```python
from build123d import *

# Parameters (mm, degrees)
F1_DEPTH = 14.37
F0_R     = 2
F2_DEPTH = 7.185
F3_DEPTH = 14.37


with BuildPart() as f1:
    # F0 (on Front) → F1 (new body)
    with BuildSketch(Plane.XZ):
        with BuildLine():
            Line((3.9000000034, 5.6), (2.8, 5.6))
            ThreePointArc((2.8, 5.6), (4.7798989873, 4.7798989873), (5.6, 2.8))
            ThreePointArc((5.6, 2.8), (6.0135800872, 1.3354181484), (7.1321428571, 0.3034947896))
            ThreePointArc((7.1321428571, 0.3034947896), (7.7481620558, 0.0769305381), (8.4, 0))
            Line((8.4, 0), (31.6, 0))
            ThreePointArc((31.6, 0), (32.2518379442, 0.0769305381), (32.8678571429, 0.3034947896))
            ThreePointArc((32.8678571429, 0.3034947896), (33.9864199128, 1.3354181484), (34.4, 2.8))
            ThreePointArc((34.4, 2.8), (35.2201010127, 4.7798989873), (37.2, 5.6))
            Line((37.2, 5.6), (37.2, 6.7))
            ThreePointArc((37.2, 6.7), (36.8778174593, 5.9221825407), (36.1, 5.6))
            Line((36.1, 5.6), (33.0575369646, 5.6))
            Line((33.0575369646, 5.6), (6.9424630354, 5.6))
            Line((6.9424630354, 5.6), (3.9000000034, 5.6))
        make_face()
        with BuildLine():
            ThreePointArc((35.2574998019, 7.4072435339), (34.0261653027, 6.6635182559), (33.0575369646, 5.6))
            Line((33.0575369646, 5.6), (36.1, 5.6))
            ThreePointArc((36.1, 5.6), (35.103012566, 6.2352247249), (35.2574998019, 7.4072435339))
        make_face()
        with BuildLine():
            ThreePointArc((35.2574998019, 7.4072435339), (35.103012566, 6.2352247249), (36.1, 5.6))
            ThreePointArc((36.1, 5.6), (36.8778174593, 5.9221825407), (37.2, 6.7))
            ThreePointArc((37.2, 6.7), (36.9926506427, 7.3427867688), (36.4487730361, 7.7432436768))
            ThreePointArc((36.4487730361, 7.7432436768), (35.8426991749, 7.6122483799), (35.2574998019, 7.4072435339))
        make_face()
        with BuildLine():
            ThreePointArc((4.7425001981, 7.4072435339), (4.8969874348, 6.2352247264), (3.9000000034, 5.6))
            Line((3.9000000034, 5.6), (6.9424630354, 5.6))
            ThreePointArc((6.9424630354, 5.6), (5.9738346973, 6.6635182559), (4.7425001981, 7.4072435339))
        make_face()
        with BuildLine():
            ThreePointArc((2.8, 6.7), (3.1221825419, 5.9221825395), (3.9000000034, 5.6))
            ThreePointArc((3.9000000034, 5.6), (4.8969874348, 6.2352247264), (4.7425001981, 7.4072435339))
            ThreePointArc((4.7425001981, 7.4072435339), (4.1573008251, 7.6122483799), (3.5512269639, 7.7432436768))
            ThreePointArc((3.5512269639, 7.7432436768), (3.0073493573, 7.3427867688), (2.8, 6.7))
        make_face()
        with BuildLine():
            Line((2.8, 6.7), (2.8, 5.6))
            Line((2.8, 5.6), (3.9000000034, 5.6))
            ThreePointArc((3.9000000034, 5.6), (3.1221825419, 5.9221825395), (2.8, 6.7))
        make_face()
    extrude(amount=F1_DEPTH)



with BuildPart() as f1b:
    # F0 (on Front) → F1, piece 2 (new body)
    with BuildSketch(Plane.XZ):
        with Locations((37.2, 2.8)):
            Circle(F0_R)
    extrude(amount=F1_DEPTH)


with BuildPart() as f1_1:
    add(f1.part)

    add(f1b.part)  # F2 merges F1b
    # F0 (on Front) → F2 (join)
    with BuildSketch(Plane.XZ):
        with BuildLine():
            ThreePointArc((34.4, 2.8), (35.2201010127, 0.8201010127), (37.2, 0))
            ThreePointArc((37.2, 0), (39.1798989873, 0.8201010127), (40, 2.8))
            ThreePointArc((40, 2.8), (39.1798989873, 4.7798989873), (37.2, 5.6))
            ThreePointArc((37.2, 5.6), (35.2201010127, 4.7798989873), (34.4, 2.8))
        make_face()
        with Locations((37.2, 2.8)):
            Circle(F0_R, mode=Mode.SUBTRACT)
    extrude(amount=F2_DEPTH)

    # F0 (on Front) → F3 (join)
    with BuildSketch(Plane.XZ):
        with BuildLine():
            ThreePointArc((5.6, 2.8), (4.7798989873, 0.8201010127), (2.8, 0))
            Line((2.8, 0), (6.9424630354, 0))
            ThreePointArc((6.9424630354, 0), (7.0400192842, 0.1500497232), (7.1321428571, 0.3034947896))
            ThreePointArc((7.1321428571, 0.3034947896), (6.0135800872, 1.3354181484), (5.6, 2.8))
        make_face()
        with BuildLine():
            ThreePointArc((2.8, 5.6), (0, 2.8), (2.8, 0))
            ThreePointArc((2.8, 0), (4.7798989873, 0.8201010127), (5.6, 2.8))
            ThreePointArc((5.6, 2.8), (4.7798989873, 4.7798989873), (2.8, 5.6))
        make_face()
        with Locations((2.8, 2.8)):
            Circle(F0_R, mode=Mode.SUBTRACT)
    extrude(amount=F3_DEPTH)


solid = f1_1.part
```
Geometry: final body of the model. Coordinates: model frame, mm. A direction names the side the tool comes from. Round coordinates to 2 decimals unless told otherwise and drop trailing zeros. Order: outer loops, then holes, each group sorted by start corner. A loop starts at its lowest first (then second) coordinate and runs counter-clockwise, first axis right, second up. Notation, with made-up numbers: (-20.75, 62.5) -> (-4.75, 62.5) arc R27 cw to (-4.75, 93.5) -> close; hole circle Ø7 at (21.25, -24.75). An arc over 180 degrees is marked (long way). Use one line per item in the form item = value. Start each with the question number.
1. Cut plane C-C (z = 4). Return the cut outline in (x, y) (3 decimals).
2. Draft query along Z for faces 1 (the face through (37, -7.185, 5)), 2 (the face through (2.8, -7, 6)), 3 (the face through (20, -7, 5.6)). Return one class per face: pulls with the +Z half, pulls with the -Z half, needs draft (parallel to the pull), parting line crosses it, or undercut.
3. Reachability of faces 4 (the face through (39.108, -10.727, 3.401)), 5 (the face through (7.74, -7.08, 0.08)), 6 (the face through (37.2, -7, 6)) from +Z, -Z, +X, -X, +Y, -Y: full face, straight path, thin tool, end or side. Return the list, or none.
4. Line query: probe 1 along X at (y, z) = (-1.5, 1); probe 2 along Z at (x, y) = (28, -1); probe 3 along X at (y, z) = (-10.75, 4). Output: solid intervals per line, ascending.
5. Cut plane B-B (y = -6.5). Return the cut outline in (x, z), then the cut area to 3 significant figures.
6. Cut plane D-D (z = 2). Return the cut outline in (x, y) (3 decimals), then the cut area to 3 significant figures.
7. Cut plane A-A (y = -11.25). Return the cut outline in (x, z).
8. Pin query (flat end, axial travel): pin 1 Ø0.6 at (y, z) = (-10, 6) entering from +X; pin 2 Ø3 at (x, y) = (20.5, -7) entering from +Z; pin 3 Ø3 at (x, z) = (2.8, 2.8) entering from +Y; pin 4 Ø0.6 at (y, z) = (-9.5, 6) entering from -X. Return the tip coordinate at first contact, or that it passes through.
Solution:
q1.outline = (0.27, -14.37) -> (1.2, -14.37) -> (1.2, 0) -> (0.27, 0) -> close; (4.4, -14.37) -> (34.67, -14.37) -> (34.67, -7.185) -> (35.6, -7.185) -> (35.6, -14.37) -> (38.8, -14.37) -> (38.8, -7.185) -> (39.73, -7.185) -> (39.73, 0) -> (4.4, 0) -> close
q2.face_1 = undercut
q2.face_2 = needs draft
q2.face_3 = pulls with the +Z half
q3.face_4 = -Y
q3.face_5 = -Z, +Y, -Y
q3.face_6 = +Z, +X, +Y, -Y
q4.probe_1 = 0.66 to 1.93, 3.67 to 33.74, 35.06 to 39.34
q4.probe_2 = 0 to 5.6
q4.probe_3 = 0.27 to 1.2, 4.4 to 34.67, 35.6 to 38.8
q5.outline = (2.8, 0) -> (6.94, 0) arc R5 ccw to (7.13, 0.3) arc R2.8 ccw to (8.4, 0) -> (31.6, 0) arc R2.8 ccw to (34.4, 2.8) arc R2.8 ccw (long way) to (37.2, 5.6) -> (37.2, 6.7) arc R1.1 ccw to (36.45, 7.74) arc R5 ccw to (33.06, 5.6) -> (6.94, 5.6) arc R5 ccw to (3.55, 7.74) arc R1.1 ccw to (2.8, 6.7) -> (2.8, 5.6) arc R2.8 ccw to start; hole circle Ø4 at (2.8, 2.8)
q5.area = 214 mm^2
q6.outline = (0.117, -14.37) -> (0.967, -14.37) -> (0.967, 0) -> (0.117, 0) -> close; (4.633, -14.37) -> (34.283, -14.37) -> (34.283, 0) -> (4.633, 0) -> close; (34.517, -7.185) -> (35.367, -7.185) -> (35.367, -14.37) -> (39.033, -14.37) -> (39.033, -7.185) -> (39.883, -7.185) -> (39.883, 0) -> (34.517, 0) -> close
q6.area = 503 mm^2
q7.outline = (2.8, 0) -> (6.94, 0) arc R5 ccw to (7.13, 0.3) arc R2.8 ccw to (8.4, 0) -> (31.6, 0) arc R2.8 ccw to (34.4, 2.8) arc R2.8 cw to (37.2, 5.6) -> (37.2, 6.7) arc R1.1 ccw to (36.45, 7.74) arc R5 ccw to (33.06, 5.6) -> (6.94, 5.6) arc R5 ccw to (3.55, 7.74) arc R1.1 ccw to (2.8, 6.7) -> (2.8, 5.6) arc R2.8 ccw to start; circle Ø4 at (37.2, 2.8); hole circle Ø4 at (2.8, 2.8)
q8.pin_1 = 37.2
q8.pin_2 = 5.6
q8.pin_3 = through
q8.pin_4 = 2.8
